Source: CAD feature listing. Evaluate the final solid. Frame: model axes, mm. A direction names the side the tool comes from. Coordinates: 2 decimals unless noted, no trailing zeros. Order: outer loops, then holes, each group sorted by start corner. A loop starts at its lowest first (then second) coordinate and runs counter-clockwise, first axis right, second up. Notation, with made-up numbers: (85, 13.25) -> (90, 13.25) arc R15 ccw to (90, 34.25) -> close; hole circle Ø10 at (-9, 61.5). An arc over 180 degrees is marked (long way). Write each question's results on one line, items separated by ' | '. Start each with the question number.
from build123d import *

# Parameters (mm, degrees)
SKETCH_1_W          = 24
SKETCH_1_H          = 40
SKETCH_1_R          = 2
EXTRUDE_1_DEPTH     = 5
EXTRUDE_5_DEPTH     = 98
SKETCH_10_W         = 10
SKETCH_10_H         = 28
EXTRUDE_6_DEPTH     = 18.5
SKETCH_12_R         = 2
CUT_EXTRUDE_4_DEPTH = 24.5
SKETCH_13_W         = 12
SKETCH_13_H         = 28
CUT_EXTRUDE_5_DEPTH = 2


with BuildPart() as part:
    # 草图1 → 凸台-拉伸1 (new body)
    with BuildSketch(Plane(origin=(0, 0, 0), x_dir=(1, 0, 0), z_dir=(0, 1, 0))):
        Rectangle(SKETCH_1_W, SKETCH_1_H)
        with Locations((7.5, -14.8)):
            Circle(SKETCH_1_R, mode=Mode.SUBTRACT)
        with Locations((-7.5, -14.8)):
            Circle(SKETCH_1_R, mode=Mode.SUBTRACT)
        with Locations((-7.5, 14.8)):
            Circle(SKETCH_1_R, mode=Mode.SUBTRACT)
        with Locations((7.5, 14.8)):
            Circle(SKETCH_1_R, mode=Mode.SUBTRACT)
    extrude(amount=EXTRUDE_1_DEPTH)

    # 草图8 → 凸台-拉伸5 (add)
    with BuildSketch(Plane(origin=(0, 5, 0), x_dir=(1, 0, 0), z_dir=(0, 1, 0))):
        Polygon((-5, 0), (-5, -20), (5, -20), (5, 20), (-5, 20), align=None)
    extrude(amount=EXTRUDE_5_DEPTH)

    # 草图10 → 凸台-拉伸6 (add)
    with BuildSketch(Plane(origin=(5, 0, 0), x_dir=(0, 0, -1), z_dir=(1, 0, 0))):
        with Locations((0, 89)):
            Rectangle(SKETCH_10_W, SKETCH_10_H)
    extrude(amount=EXTRUDE_6_DEPTH)

    # 草图12 → 切除-拉伸4 (cut)
    with BuildSketch(Plane(origin=(0, 0, -5), x_dir=(-1, 0, 0), z_dir=(0, 0, -1))):
        with Locations((-15.41, 98.67)):
            Circle(SKETCH_12_R)
        with Locations((-15.41, 88.85)):
            Circle(SKETCH_12_R)
        with Locations((-15.41, 79.03)):
            Circle(SKETCH_12_R)
    extrude(amount=-CUT_EXTRUDE_4_DEPTH, mode=Mode.SUBTRACT)

    # 草图13 → 切除-拉伸5 (cut, symmetric)
    with BuildSketch(Plane.XY):
        with Locations((17.5, 89)):
            Rectangle(SKETCH_13_W, SKETCH_13_H)
    extrude(amount=CUT_EXTRUDE_5_DEPTH, both=True, mode=Mode.SUBTRACT)


solid = part.part
(1) Reachability of faces 5 (the flat face through (11.5, 89, 0)), 6 (the flat face through (12, 2, 0)), 7 (the flat face through (8, 5, 0)) from +Z, -Z, +X, -X, +Y, -Y: full face, straight path, thin tool, end or side. Return the list, or none.
(2) Section B-B on x = 7.5. Return the cut outline in (y, z), then the cut area to 3 significant figures.
(3) Section A-A on z = -14.8. Return the cut outline in (x, y), then the cut area to 3 significant figures.
(4) First-contact query: P1, Ø4, axis at x = 15.5, z = -8, coming from the +Y side; P2, Ø5.5, axis at x = 18, y = 86, coming from the -Z side; P3, Ø13, axis at x = 15.5, y = 85.5, coming from the +Z side; P4, Ø3.5, axis at x = -8.5, z = -4, coming from the +Y side. Flat tips, straight axial feed; report the tip coordinate or a pass-through.
(5) Draft query along Y for faces 1 (the flat face through (0, 0, 0)), 2 (the flat face through (-9, 5, 0)), 3 (the cylindrical face through (15.844, 86.898, 3.479)), 4 (the cylindrical face through (5.9, 2.5, -13.6)). Return one class per face: released by +Y, released by -Y, zero draft, split by the parting line, or undercut.
(6) Section D-D on x = 20. Return the cut outline in (y, z).
(7) Section C-C on y = 79.03. Return the cut outline in (x, z).
(8) Line query: L1, parallel to Z at x = 7.5, y = 2.5; L2, parallel to Y at x = 15.41, z = -2.65; L3, parallel to Z at x = 7, y = 2. Output: solid intervals per line, ascending.
Results list:
1) face 5: +X, +Y | face 6: +Z, -Z, +X, -Y | face 7: +Z, -Z, +X
2) outline: (0, -20) -> (5, -20) -> (5, -16.8) -> (0, -16.8) -> close; (0, -12.8) -> (5, -12.8) -> (5, 12.8) -> (0, 12.8) -> close; (0, 16.8) -> (5, 16.8) -> (5, 20) -> (0, 20) -> close; (75, -5) -> (103, -5) -> (103, 5) -> (75, 5) -> close | area: 440 mm²
3) outline: (-12, 0) -> (-9.5, 0) -> (-9.5, 5) -> (-12, 5) -> close; (-5.5, 0) -> (5.5, 0) -> (5.5, 5) -> (5, 5) -> (5, 103) -> (-5, 103) -> (-5, 5) -> (-5.5, 5) -> close; (9.5, 0) -> (12, 0) -> (12, 5) -> (9.5, 5) -> close | area: 1,060 mm²
4) P1: passes through | P2: stops at z = -5 | P3: stops at z = 5 | P4: stops at y = 5
5) face 1: released by -Y | face 2: released by +Y | face 3: undercut | face 4: zero draft
6) outline: (75, -5) -> (103, -5) -> (103, -2) -> (75, -2) -> close; (75, 2) -> (103, 2) -> (103, 5) -> (75, 5) -> close
7) outline: (-5, -20) -> (5, -20) -> (5, -5) -> (13.41, -5) -> (13.41, -2) -> (11.5, -2) -> (11.5, 2) -> (13.41, 2) -> (13.41, 5) -> (5, 5) -> (5, 20) -> (-5, 20) -> close; (17.41, -5) -> (23.5, -5) -> (23.5, -2) -> (17.41, -2) -> close; (17.41, 2) -> (23.5, 2) -> (23.5, 5) -> (17.41, 5) -> close
8) L1: z = -20 to -16.8, -12.8 to 12.8, 16.8 to 20 | L2: y = 75 to 77.03, 81.03 to 86.85, 90.85 to 96.67, 100.67 to 103 | L3: z = -20 to -16.74, -12.86 to 12.86, 16.74 to 20
